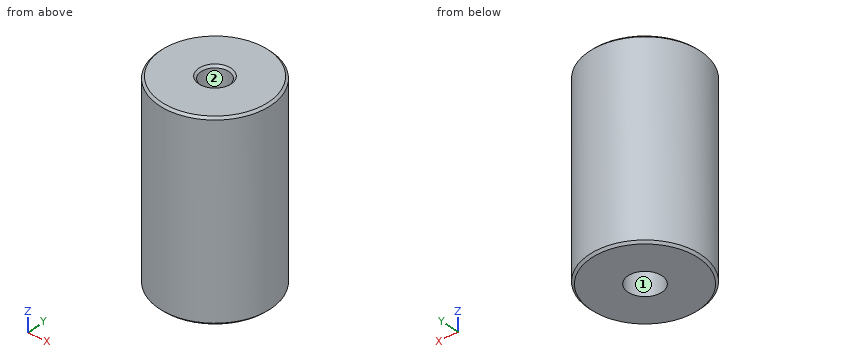
```python
from build123d import *

# Parameters (mm, degrees)
SKETCH1_R                          = 12.7
BOSS_EXTRUDE1_DEPTH                = 43.6
SKETCH2_R                          = 3.1877
CUT_EXTRUDE1_DEPTH                 = 48.154427152
F_5_16_0_3125_DIAMETER_HOLE1_D     = 7.71652
F_5_16_0_3125_DIAMETER_HOLE1_DEPTH = 18.796
F_5_16_0_3125_DIAMETER_HOLE1_TIP   = 2.318276492
CHAMFER1_SIZE                      = 0.5
CHAMFER2_SIZE                      = 0.5


with BuildPart() as part:
    # Sketch1 → Boss-Extrude1 (new body)
    with BuildSketch(Plane.XY):
        Circle(SKETCH1_R)
    extrude(amount=BOSS_EXTRUDE1_DEPTH)

    # Sketch2 → Cut-Extrude1 (cut, through all)
    with BuildSketch(Plane.XY.offset(43.6)):
        Circle(SKETCH2_R)
    extrude(amount=-CUT_EXTRUDE1_DEPTH, mode=Mode.SUBTRACT)

    # 5/16 (0.3125) Diameter Hole1
    with Locations(Plane(origin=(0, 0, 0), x_dir=(-1, 0, 0), z_dir=(0, 0, -1))):
        with Locations((0, 0)):
            Hole(F_5_16_0_3125_DIAMETER_HOLE1_D / 2, depth=F_5_16_0_3125_DIAMETER_HOLE1_DEPTH)
            with Locations((0, 0, -(F_5_16_0_3125_DIAMETER_HOLE1_DEPTH + F_5_16_0_3125_DIAMETER_HOLE1_TIP / 2))):  # 118° drill point
                Cone(0, F_5_16_0_3125_DIAMETER_HOLE1_D / 2, F_5_16_0_3125_DIAMETER_HOLE1_TIP, mode=Mode.SUBTRACT)

    # Chamfer1
    chamfer1_edges = [part.edges().sort_by_distance(p)[0] for p in [
        (-12.7, 0, 0),
        (-12.7, 0, 43.6),
    ]]
    chamfer(chamfer1_edges, length=CHAMFER1_SIZE)

    # Chamfer2
    chamfer2_edges = [part.edges().sort_by_distance(p)[0] for p in [
        (-3.1877, 0, 43.6),
    ]]
    chamfer(chamfer2_edges, length=CHAMFER2_SIZE)


solid = part.part
```
Input: part model. Units: mm. Frame: model coordinates. Face numbers are marked on the shaded views. A direction names the side the tool comes from. Round coordinates to 2 decimals unless told otherwise and drop trailing zeros. Write each loop counter-clockwise with the first axis right and the second up, starting at its lowest first coordinate (ties: lowest second). Pieces come first, ordered by that corner, then holes. Notation, with made-up numbers: (67, -4.75) - (97, -4.75) arc R8 ccw to (97, 4.25) - close; hole circle Ø5 at (46, 50.5). An arc over 180 degrees is marked (long way). Write item = value, one per line.
(1) Material intervals for probe 1 along Y at (x, z) = (0, 37); probe 2 along Y at (x, z) = (0, 9.25); probe 3 along X at (y, z) = (2, 21), sorted ascending.
Geometry check:
probe_1 = -12.7 to -3.19, 3.19 to 12.7
probe_2 = -12.7 to -3.86, 3.86 to 12.7
probe_3 = -12.54 to -2.48, 2.48 to 12.54
(2) Section query D-D on z = 28. Output: boundary loops of the cut face in (x, y), then the cut area to 3 significant figures.
Geometry check:
outline = circle Ø25.4 at (0, 0); hole circle Ø6.38 at (0, 0)
area = 475 mm^2
(3) Contact query for flat-ended pins moving along their axis: pin 1 Ø2 at (y, z) = (-1.5, 24.5) entering from +X; pin 2 Ø7 at (x, y) = (0, 0) entering from -Z; pin 3 Ø1.5 at (y, z) = (7.5, 14) entering from -X. Output: stop coordinate, or through.
Geometry check:
pin_1 = 12.69
pin_2 = 19.01
pin_3 = -10.76
(4) Section query A-A on y = 0. Output: boundary loops of the cut face in (x, z).
Geometry check:
outline = (-12.7, 0.5) - (-12.2, 0) - (-3.86, 0) - (-3.86, 18.8) - (-3.19, 19.2) - (-3.19, 43.1) - (-3.69, 43.6) - (-12.2, 43.6) - (-12.7, 43.1) - close; (3.19, 19.2) - (3.86, 18.8) - (3.86, 0) - (12.2, 0) - (12.7, 0.5) - (12.7, 43.1) - (12.2, 43.6) - (3.69, 43.6) - (3.19, 43.1) - close
(5) Access query for the marked faces 1 and 2. Directions: +Z, -Z, +X, -X, +Y, -Y. A direction counts if a zero-diameter tool reaches every point of the face in a straight line with its end or side. Return the directions, or none.
Geometry check:
face_1 = -Z
face_2 = +Z, -Z
(6) Section query C-C on z = 15.5. Output: boundary loops of the cut face in (x, y), then the cut area to 3 significant figures.
Geometry check:
outline = circle Ø25.4 at (0, 0); hole circle Ø7.72 at (0, 0)
area = 460 mm^2
